Source: CAD feature listing. Evaluate the final solid. Frame: model axes, mm. Round coordinates to 2 decimals unless told otherwise and drop trailing zeros. Loops run counter-clockwise (first coordinate to the right, second up) from the corner with the lowest first, then second, coordinate; pieces in that order, holes last. Notation, with made-up numbers: (-17.75, -15.5) - (13.25, -15.5) arc R15 ccw to (13.25, 9.5) - close; hole circle Ø1 at (34, 12). An arc over 180 degrees is marked (long way). One line per question, with ' | ' between items.
from build123d import *

# Parameters (mm, degrees)
SKETCH1_R           = 2.5
SKETCH1_R_2         = 10
BOSS_EXTRUDE1_DEPTH = 1
SKETCH2_R           = 1.5
CUT_EXTRUDE1_DEPTH  = 230.926075076
FILLET1_R           = 0.5
FILLET2_R           = 10
CUT_EXTRUDE2_DEPTH  = 10
FILLET3_R           = 2
FILLET4_R           = 0.5


with BuildPart() as part:
    # Sketch1 → Boss-Extrude1 (new body)
    with BuildSketch(Plane.XY):
        Polygon((0, 0), (76, 0), (76, 217), (-12.55, 217), (-12.55, 212), (-19.55, 212), (-19.55, 217), (-32, 217), (-32, 175), (0, 175), align=None)
        with Locations((14, 169.15)):
            Circle(SKETCH1_R, mode=Mode.SUBTRACT)
        with Locations((14, 10.85)):
            Circle(SKETCH1_R, mode=Mode.SUBTRACT)
        with Locations((64, 10.85)):
            Circle(SKETCH1_R, mode=Mode.SUBTRACT)
        with Locations((64, 211.15)):
            Circle(SKETCH1_R, mode=Mode.SUBTRACT)
        with Locations((18, 196)):
            Circle(SKETCH1_R_2, mode=Mode.SUBTRACT)
        with BuildLine():
            Line((-19.55, 207), (-12.55, 207))
            ThreePointArc((-12.55, 207), (-11.425, 205.875), (-12.55, 204.75))
            Line((-12.55, 204.75), (-19.55, 204.75))
            ThreePointArc((-19.55, 204.75), (-20.675, 205.875), (-19.55, 207))
        make_face(mode=Mode.SUBTRACT)
    extrude(amount=BOSS_EXTRUDE1_DEPTH)

    # Sketch2 → Cut-Extrude1 (cut, through all)
    with BuildSketch(Plane.XY.offset(1)):
        with Locations((-13.610660172, 213.060660172)):
            Circle(SKETCH2_R)
        with Locations((-18.489339828, 213.060660172)):
            Circle(SKETCH2_R)
    extrude(amount=-CUT_EXTRUDE1_DEPTH, mode=Mode.SUBTRACT)

    # Fillet1
    fillet1_edges = [part.edges().sort_by_distance(p)[0] for p in [
        (-32, 217, 0.5),
        (-19.55, 217, 0.5),
        (-12.55, 217, 0.5),
        (76, 217, 0.5),
        (76, 0, 0.5),
        (0, 0, 0.5),
    ]]
    fillet(fillet1_edges, radius=FILLET1_R)

    # Fillet2
    fillet2_edges = [part.edges().sort_by_distance(p)[0] for p in [
        (0, 175, 0.5),
        (-32, 175, 0.5),
    ]]
    fillet(fillet2_edges, radius=FILLET2_R)

    # Sketch4 → Cut-Extrude2 (cut)
    with BuildSketch(Plane.XY.offset(1)):
        with BuildLine():
            Line((-2, 217), (-2, 171))
            ThreePointArc((-2, 171), (-5.865545946, 173.268908108), (-10, 175))
            Line((-10, 175), (-22, 175))
            ThreePointArc((-22, 175), (-29.071067812, 177.928932188), (-32, 185))
            Line((-32, 185), (-32, 216.5))
            ThreePointArc((-32, 216.5), (-31.853553391, 216.853553391), (-31.5, 217))
            Line((-31.5, 217), (-20.05, 217))
            ThreePointArc((-20.05, 217), (-19.696446609, 216.853553391), (-19.55, 216.5))
            Line((-19.55, 216.5), (-19.55, 214.121320344))
            ThreePointArc((-19.55, 214.121320344), (-19.55, 212), (-17.428679656, 212))
            Line((-17.428679656, 212), (-14.671320344, 212))
            ThreePointArc((-14.671320344, 212), (-12.55, 212), (-12.55, 214.121320344))
            Line((-12.55, 214.121320344), (-12.55, 216.5))
            ThreePointArc((-12.55, 216.5), (-12.403553391, 216.853553391), (-12.05, 217))
            Line((-12.05, 217), (-2, 217))
        make_face()
    extrude(amount=-CUT_EXTRUDE2_DEPTH, mode=Mode.SUBTRACT)

    # Fillet3
    fillet3_edges = [part.edges().sort_by_distance(p)[0] for p in [
        (-2, 171, 0.5),
    ]]
    fillet(fillet3_edges, radius=FILLET3_R)

    # Fillet4
    fillet4_edges = [part.edges().sort_by_distance(p)[0] for p in [
        (-2, 217, 0.5),
    ]]
    fillet(fillet4_edges, radius=FILLET4_R)


solid = part.part
1. Mould query, pull axis Y, two halves, no side actions, for faces 1 (the flat face through (36, 110, 1)), 2 (the cylindrical face through (15.83, 186.24, 0.49)). Classes: released by +Y, released by -Y, zero draft, split by the parting line, or undercut.
Worked out:
face 1: zero draft | face 2: undercut
2. Material intervals for probe 1 along X at (y, z) = (10.5, 0.3); probe 2 along Y at (x, z) = (18, 0.5); probe 3 along Y at (x, z) = (64, 0.6), sorted ascending.
Worked out:
probe 1: x = 0 to 11.52, 16.48 to 61.52, 66.48 to 76 | probe 2: y = 0 to 186, 206 to 217 | probe 3: y = 0 to 8.35, 13.35 to 208.65, 213.65 to 217
3. Section query B-B, the plane x = 64. Return loops of the section in (y, z).
Worked out:
outline: (0, 0) - (8.35, 0) - (8.35, 1) - (0, 1) - close; (13.35, 0) - (208.65, 0) - (208.65, 1) - (13.35, 1) - close; (213.65, 0) - (217, 0) - (217, 1) - (213.65, 1) - close
4. Section query C-C, the plane y = 10.85. Return loops of the section in (x, z).
Worked out:
outline: (0, 0) - (11.5, 0) - (11.5, 1) - (0, 1) - close; (16.5, 0) - (61.5, 0) - (61.5, 1) - (16.5, 1) - close; (66.5, 0) - (76, 0) - (76, 1) - (66.5, 1) - close
5. Section query A-A, the plane y = 196. Return loops of the section in (x, z), plus the area to 3 significant figures.
Worked out:
outline: (-2, 0) - (8, 0) - (8, 1) - (-2, 1) - close; (28, 0) - (76, 0) - (76, 1) - (28, 1) - close | area: 58.0 mm2
6. Section query D-D, the plane z = 0.5. Return loops of the section in (x, y), plus the area to 3 significant figures.
Worked out:
outline: (-2, 171.63) arc R2 ccw to (-1.67, 170.53) arc R10 cw to (0, 165) - (0, 0.5) arc R0.5 ccw to (0.5, 0) - (75.5, 0) arc R0.5 ccw to (76, 0.5) - (76, 216.5) arc R0.5 ccw to (75.5, 217) - (-1.5, 217) arc R0.5 ccw to (-2, 216.5) - close; hole circle Ø20 at (18, 196); hole circle Ø5 at (14, 10.85); hole circle Ø5 at (14, 169.15); hole circle Ø5 at (64, 10.85); hole circle Ø5 at (64, 211.15) | area: 16,200 mm2
7. Contact query for a flat-ended pin moving along its axis: P1, Ø4, axis at x = 14, y = 10.85, coming from the +Z side. Output: stop coordinate, or through.
Worked out:
P1: passes through
